Autodesk Inventor part; units mm, degrees
ref_plane "YZ Plane" through (0, 0, 0) normal (1, 0, 0) x (0, 1, 0)
ref_plane "XZ Plane" through (0, 0, 0) normal (0, 1, 0) x (-1, 0, 0)
ref_plane "XY Plane" through (0, 0, 0) normal (0, 0, 1) x (1, 0, 0)
sketch "Sketch1" plane through (0, 0, 0) normal (0, 0, 1) x (1, 0, 0)
  line L0 (-27.9942, -0.0006) -> (-27.9942, -3.8862)
  line L1 (-27.9942, -3.8862) -> (-31.22, -3.8862)
  line L2 (27.7334, 0) -> (27.7334, -3.8862)
  line L3 (-31.22, -3.8862) -> (-31.22, 45.0041)
  line L4 (27.7334, -3.8862) -> (30.9592, -3.8862)
  line L5 (30.9592, -3.8862) -> (30.9592, 45.0041)
  line L6 (30.9592, 45.0041) -> (-31.22, 45.0041)
  line L7 (27.7334, -3.8862) -> (27.7334, 0)
  line L8 (27.7334, 0) -> (27.7334, 6.9041)
  line L9 (27.7334, 6.9041) -> (-27.9942, 6.9041)
  line L10 (-27.9942, 6.9041) -> (-27.9942, -0.0006)
  line L11 (30.9592, 6.9041) -> (-31.22, 6.9041)
  point P0 (0, 0)
  point P1 (27.7334, 4.1367)
  dimension "d3" = 3.2258
  dimension "d4" = 55.7276
  dimension "d5" = 3.2258
  dimension "d33" = 38.1
extrude "Extrusion1" add sketch "Sketch1" along normal blind 3.2258
sketch "Sketch2" plane through (30.9592, -3.8862, 0) normal (1, 0, 0) x (0, 0, -1)
  point P0 (0, 3.8862)
sketch "Sketch4" plane through (0, 0, 0) normal (0, 0, -1) x (-1, 0, 0)
  point P0 (0, 0)
sketch "Sketch5" plane through (0, 0, 0) normal (0, 0, -1) x (-1, 0, 0)
  line L0 (-30.9592, -3.8862) -> (-30.9592, 45.0041)
  line L1 (-30.9592, 0) -> (-30.9592, -1.27)
  line L2 (-30.9592, 0) -> (-32.2292, 0)
  line L3 (-32.2292, 0) -> (-32.2292, 45.0041)
  line L4 (-32.2292, 45.0041) -> (-30.9592, 45.0041)
  line L5 (-30.9592, 45.0041) -> (31.22, 45.0041)
  line L6 (0.1304, 45.0041) -> (0.1304, 20.6375)
  line L7 (31.22, 0) -> (32.49, 0)
  line L8 (32.49, 0) -> (32.49, 45.0041)
  line L9 (32.49, 45.0041) -> (31.22, 45.0041)
  line L10 (31.22, 45.0041) -> (31.22, -3.8862)
  point P0 (0, 0)
  point P1 (-21.0964, 42.2367)
  point P2 (21.0964, 42.2367)
  point P3 (31.22, 0)
  dimension "d14" = 1.27
  dimension "d15" = 1.27
extrude "Extrusion3" add sketch "Sketch5" against normal blind 3.2258
sketch "Sketch10" plane through (0, 0, 0) normal (0, 0, -1) x (-1, 0, 0)
  point P0 (0, 0)
sketch "Sketch11" plane through (0, 0, 0) normal (0, 0, -1) x (-1, 0, 0)
  point P0 (0, 0)
sketch "Sketch13" plane through (0, 0, 0) normal (0, 0, -1) x (-1, 0, 0)
  line L0 (-32.2292, 45.0041) -> (-32.2292, 0)
  line L1 (-32.2292, 45.0041) -> (27.4604, 45.0041) construction
  line L2 (-56.5071, -9.525) -> (-32.8958, -9.525)
  line L3 (-32.2292, 0) -> (-30.9592, 0)
  line L4 (-32.2292, 0) -> (-32.2292, -9.525)
  line L5 (-32.2292, -9.525) -> (-32.8958, -9.525)
  line L6 (-34.925, 46.2044) -> (-32.2292, 45.0041)
  line L7 (-59.2029, -8.3247) -> (-56.5071, -9.525)
  line L8 (-56.5071, -2.2699) -> (-53.8113, -3.4701)
  line L9 (-53.8113, 3.175) -> (-51.3422, 2.0757)
  line L10 (-37.1197, 41.275) -> (-34.4239, 40.0747)
  line L11 (-36.0254, 36.4778) -> (-38.7212, 37.678)
  line L12 (-38.4353, 31.0649) -> (-41.1312, 32.2651)
  line L13 (-34.925, 46.2044) -> (-37.1197, 41.275)
  line L14 (-38.7212, 37.678) -> (-41.1312, 32.2651)
  line L15 (-56.5071, -2.2699) -> (-59.2029, -8.3247)
  line L16 (-51.2557, 9.525) -> (-48.5599, 8.3247)
  line L17 (-59.2029, -8.3247) -> (-56.5071, -2.2699)
  line L18 (-53.8113, 3.175) -> (-54.038, 3.2759)
  line L19 (-56.5071, -2.2699) -> (-59.2029, -8.3247)
  line L20 (-49.5406, 13.3771) -> (-46.8448, 12.1769)
  line L21 (-47.0149, 19.05) -> (-44.3682, 17.7396)
  line L22 (-45.478, 22.5021) -> (-42.7821, 21.3018)
  line L23 (-43.4768, 26.9966) -> (-40.781, 25.7964)
  line L24 (-34.925, 46.2044) -> (-37.1197, 41.275)
  line L25 (-38.7212, 37.678) -> (-41.1312, 32.2651)
  line L26 (-49.5406, 13.3771) -> (-47.0149, 19.05)
  line L27 (-45.478, 22.5021) -> (-43.4768, 26.9966)
  line L28 (-47.0149, 19.05) -> (-49.5406, 13.3771)
  line L29 (-51.2557, 9.525) -> (-54.038, 3.2759)
  line L30 (-51.3422, 2.0757) -> (-53.8113, -3.4701)
  line L31 (-46.8448, 12.1769) -> (-48.5599, 8.3247)
  line L32 (-42.7821, 21.3018) -> (-44.3682, 17.7396)
  line L33 (-34.4239, 40.0747) -> (-36.0254, 36.4778)
  line L34 (-38.4353, 31.0649) -> (-40.781, 25.7964)
  point P0 (0, 0)
extrude "Extrusion8" add sketch "Sketch13" against normal blind 3.2258
sketch "Sketch14" plane through (0, 0, 3.2258) normal (0, 0, 1) x (1, 0, 0)
  line L0 (-32.49, 45.0041) -> (32.2292, 45.0041)
  line L1 (-23.0867, 39.6875) -> (-23.0867, 31.75)
  line L2 (23.8125, 31.75) -> (23.8125, 39.6875)
  line L3 (-23.0867, 31.75) -> (-23.0867, 28.575)
  line L4 (23.8125, 28.575) -> (23.8125, 31.75)
  line L5 (-23.0867, 39.6875) -> (23.8125, 39.6875)
  line L6 (-23.0867, 28.575) -> (-23.0867, 20.6375)
  line L7 (-23.0867, 20.6375) -> (23.8125, 20.6375)
  line L8 (23.8125, 20.6375) -> (23.8125, 28.575)
  point P0 (0, 0)
  point P1 (-27.9942, 45.0041)
  point P2 (27.7334, 45.0041)
extrude "Extrusion9" cut sketch "Sketch14" against normal through all
sketch "Sketch15" plane through (0, 0, 0) normal (0, 0, -1) x (-1, 0, 0)
  line L0 (27.9942, 6.9041) -> (-27.7334, 6.9041)
  line L1 (-27.7334, 6.9041) -> (-27.7334, 8.7347)
  line L2 (-27.7334, 8.7347) -> (27.9942, 8.7347)
  line L3 (27.9942, 8.7347) -> (27.9942, 6.9041)
  point P0 (0, 0)
extrude "Extrusion10" cut sketch "Sketch15" against normal through all
sketch "Sketch16" plane through (0, 0, 3.2258) normal (0, 0, 1) x (1, 0, 0)
  line L0 (37.1197, 41.275) -> (34.4239, 40.0747)
  line L1 (34.4239, 40.0747) -> (29.6487, 50.8)
  line L2 (34.4239, 40.0747) -> (46.1641, 40.0747) construction
  line L3 (-32.49, 45.0041) -> (-32.49, 0)
  line L4 (-32.49, 45.0041) -> (-32.49, 60.9185)
  line L5 (-32.49, 60.9185) -> (25.1436, 60.9185)
  line L6 (25.1436, 60.9185) -> (29.6487, 50.8)
  line L7 (-32.49, 45.0041) -> (32.2292, 45.0041)
  line L8 (-32.49, 45.0041) -> (32.2292, 45.0041)
  line L9 (-31.22, 48.8903) -> (-31.22, 45.0041)
  line L10 (-31.22, 45.0041) -> (-31.22, 48.8903)
  line L11 (-31.22, 48.8903) -> (-28.575, 48.8903)
  line L12 (-31.22, 48.8903) -> (-27.9942, 48.8903)
  line L13 (-27.9942, 48.8903) -> (-27.9942, 45.0041)
  line L14 (-27.9942, 48.8903) -> (-27.9942, 45.0041)
  line L15 (-32.49, 45.0041) -> (32.2292, 45.0041)
  line L16 (27.7334, 45.0041) -> (27.7334, 48.8903)
  line L17 (27.7334, 45.0041) -> (27.7334, 48.8903)
  line L18 (27.7334, 48.8903) -> (30.9592, 48.8903)
  line L19 (27.7334, 48.8903) -> (30.9592, 48.8903)
  line L20 (-29.187, 48.8903) -> (-27.9942, 48.8903)
  line L21 (32.2292, 45.0041) -> (34.925, 46.2044)
  line L22 (-32.49, 45.0041) -> (32.2292, 45.0041)
  line L23 (25.1436, 60.9185) -> (32.2292, 45.0041)
  point P0 (0, 0)
  point P1 (30.9592, 45.0041)
  dimension "d47" = 114
sketch "Sketch17" plane through (0, 0, 3.2258) normal (0, 0, 1) x (1, 0, 0)
  line L0 (-32.49, 45.0041) -> (32.2292, 45.0041)
  line L1 (-32.49, 45.0041) -> (32.2292, 45.0041)
  point P0 (0, 0)
extrude "Extrusion11" add sketch "Sketch16" against normal blind 3.2258
properties part number "mcdave_rail2"
Design review of the part built by this model. Coordinates are the model's own, in mm. A direction names the side the tool comes from. Give positions to 0.01 mm unless a question says otherwise; leave off trailing zeros. Write each loop counter-clockwise with the first axis right and the second up, starting at its lowest first coordinate (ties: lowest second). Pieces come first, ordered by that corner, then holes.
(1) Tool access review of faces 1 (the face through (36.01, 43.77, 1.59)), 2 (the face through (43.56, 19.55, 1.59)), 3 (the face through (30.959, -2, 2)): name each direction out of +Z, -Z, +X, -X, +Y, -Y from which nothing blocks a thin tool from reaching the whole face with its end or side.
Checked values:
face 1: +Z, -Z, +X, +Y
face 2: +Z, -Z
face 3: +Z, -Z, -Y
(2) Add section C-C (y = 53.5). Give the boundary of the cut face in (x, z).
Checked values:
outline: (-32.49, 0) - (28.45, 0) - (28.45, 3.23) - (-32.49, 3.23) - close
(3) Add section D-D (y = 14.5). Give the boundary of the cut face in (x, z).
Checked values:
outline: (-32.49, 0) - (49.04, 0) - (49.04, 3.23) - (-32.49, 3.23) - close
(4) Clearance check with flat-ended pins moving along their axes: pin 1 Ø6 at (x, y) = (42, 13) entering from -Z; pin 2 Ø1 at (y, z) = (4.5, 1.5) entering from +X; pin 3 Ø1.6 at (x, z) = (12, 2) entering from -Y; pin 4 Ø1 at (y, z) = (-2.5, 1) entering from -X. State where each tip first meets the part, or that it passes through.
Checked values:
pin 1: stops at z = 0
pin 2: stops at x = 53.72
pin 3: stops at y = 8.73
pin 4: stops at x = -31.22
(5) Mouldability with a two-part tool opening along X and no side actions: class faces 4 (the face through (42.148, 26.405, 1.59)), 5 (the face through (48.212, 12.785, 1.59)), 6 (the face through (47.69, 10.28, 1.59)), 7 (the face through (-4, 60.918, 2)) as +X half, -X half, draft (parallel to the pull), parting line (faces both ways), or undercut.
Checked values:
face 4: undercut
face 5: +X half
face 6: undercut
face 7: draft
(6) Wall thickness on line 1 along Y through (x, z) = (-10, 2.3); line 2 along X through (y, z) = (1.5, 1.3); line 3 along Y through (x, z) = (48.5, 1.4) (3 decimals): over which ranges is each line inside the solid? List them lowest first.
Checked values:
line 1: y = 8.73 to 20.64, 39.69 to 60.92
line 2: x = -32.49 to -27.99, 27.73 to 51.6
line 3: y = -9.525 to 8.459, 12.914 to 15.714
(7) Add section A-A (x = -7.5). Give the boundary of the cut face in (y, z), and give its area (3 significant figures).
Checked values:
outline: (8.73, 0) - (20.64, 0) - (20.64, 3.23) - (8.73, 3.23) - close; (39.69, 0) - (60.92, 0) - (60.92, 3.23) - (39.69, 3.23) - close
area: 107 mm2
(8) Add section B-B (y = 29). Give the boundary of the cut face in (x, z).
Checked values:
outline: (-32.49, 0) - (-23.09, 0) - (-23.09, 3.23) - (-32.49, 3.23) - close; (23.81, 0) - (39.35, 0) - (39.35, 3.23) - (23.81, 3.23) - close
